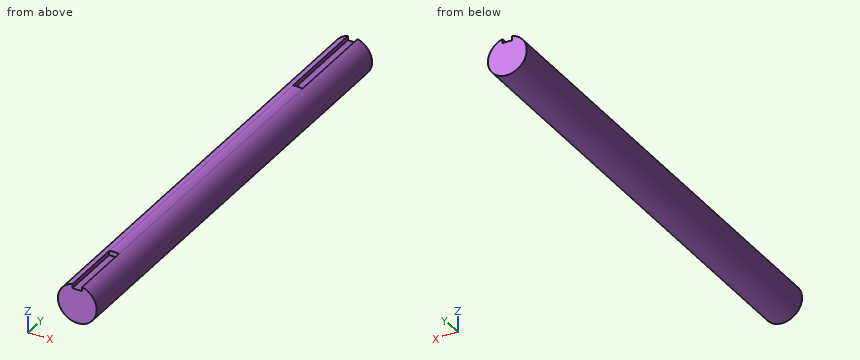
from build123d import *

# Parameters (mm, degrees)
F1_DEPTH = 762
F2_DEPTH = 152.4
F4_DEPTH = 101.6


with BuildPart() as f1:
    # F0 (on Front) → F1 (new body)
    with BuildSketch(Plane.XZ):
        with BuildLine():
            ThreePointArc((-7.9375, 30.741805), (-19.442825, -25.100579), (31.75, 0))
            ThreePointArc((31.75, 0), (25.100579, 19.442825), (7.9375, 30.741805))
            Line((7.9375, 30.741805), (7.9375, 23.8125))
            Line((7.9375, 23.8125), (-7.9375, 23.8125))
            Line((-7.9375, 23.8125), (-7.9375, 30.741805))
        make_face()
        with BuildLine():
            Line((7.9375, 23.8125), (7.9375, 30.741805))
            ThreePointArc((7.9375, 30.741805), (0, 31.75), (-7.9375, 30.741805))
            Line((-7.9375, 30.741805), (-7.9375, 23.8125))
            Line((-7.9375, 23.8125), (7.9375, 23.8125))
        make_face()
    extrude(amount=F1_DEPTH)

    # F0 (on Front) → F2 (cut)
    with BuildSketch(Plane.XZ):
        with BuildLine():
            Line((7.9375, 23.8125), (7.9375, 30.741805))
            ThreePointArc((7.9375, 30.741805), (0, 31.75), (-7.9375, 30.741805))
            Line((-7.9375, 30.741805), (-7.9375, 23.8125))
            Line((-7.9375, 23.8125), (7.9375, 23.8125))
        make_face()
    extrude(amount=F2_DEPTH, mode=Mode.SUBTRACT)

    # F3 (on face) → F4 (cut)
    with BuildSketch(Plane.XZ.offset(762)):
        with BuildLine():
            Line((-7.9375, 23.8125), (7.9375, 23.8125))
            Line((7.9375, 23.8125), (7.9375, 30.741805))
            ThreePointArc((7.9375, 30.741805), (0, 31.75), (-7.9375, 30.741805))
            Line((-7.9375, 30.741805), (-7.9375, 23.8125))
        make_face()
    extrude(amount=-F4_DEPTH, mode=Mode.SUBTRACT)


solid = f1.part
The model under review builds one solid part; all positions refer to its coordinate system, in mm. Coordinates: 2 decimals unless noted, no trailing zeros. Write each loop counter-clockwise with the first axis right and the second up, starting at its lowest first coordinate (ties: lowest second). Pieces come first, ordered by that corner, then holes. Notation, with made-up numbers: M -32.5,63 L -25.5,63 A22 cw -25.5,101 Z; hole C 79.5,76.25 d5. An arc over 180 degrees is marked long. Put each result on its own line as item: value.
1) Add section C-C on z = -20.5. Give the boundary of the cut face in (x, y), then the cut area to 3 significant figures.
Computed:
outline: M -24.24,-762 L 24.24,-762 L 24.24,0 L -24.24,0 Z
area: 36,900 mm2
2) Add section A-A on x = 0. Give the boundary of the cut face in (y, z).
Computed:
outline: M -762,-31.75 L 0,-31.75 L 0,23.81 L -152.4,23.81 L -152.4,31.75 L -660.4,31.75 L -660.4,23.81 L -762,23.81 Z
3) Clearance check with flat-ended pins moving along their axes: pin 1 Ø1 at (y, z) = (-103, -8) entering from +X; pin 2 Ø4 at (x, z) = (1, 29) entering from +Y; pin 3 Ø1 at (y, z) = (-234.5, -7) entering from -X. State where each tip first meets the part, or that it passes through.
Computed:
pin 1: stops at x = 30.85
pin 2: stops at y = -152.4
pin 3: stops at x = -31.08
4) Add section B-B on y = -683. Give the boundary of the cut face in (x, z), then the cut area to 3 significant figures.
Computed:
outline: M -7.94,23.81 L -7.94,30.74 A31.75 ccw long 31.75,0 A31.75 ccw 7.94,30.74 L 7.94,23.81 Z
area: 3,050 mm2
5) Wall thickness on probe 1 along Z at (x, y) = (0, -688); probe 2 along Y at (x, z) = (3, 28.5); probe 3 along X at (y, z) = (-107.5, 0.5): over which ranges is each line inside the solid? List them lowest first. Write a range as [from, to].
Computed:
probe 1: z = [-31.75, 23.81]
probe 2: y = [-660.4, -152.4]
probe 3: x = [-31.75, 31.75]
